from build123d import *

# Parameters (mm, degrees)
BOSS_EXTRUDE1_DEPTH = 3.175
SKETCH2_R           = 1.5875
SKETCH2_W           = 80.264
SKETCH2_H           = 12.954
CUT_EXTRUDE1_DEPTH  = 223.985606318
SKETCH7_R           = 2.032
SKETCH7_R_2         = 1.651
SKETCH7_W           = 47.244
SKETCH7_H           = 139.192
CUT_EXTRUDE4_DEPTH  = 223.985606318
SKETCH8_R           = 1.651
CUT_EXTRUDE5_DEPTH  = 223.985606318
SKETCH9_R           = 1.778
CUT_EXTRUDE6_DEPTH  = 221.482742149
CUT_EXTRUDE7_DEPTH  = 221.482742149


with BuildPart() as part:
    # Sketch1 → Boss-Extrude1 (new body)
    with BuildSketch(Plane(origin=(0, 0, 0), x_dir=(1, 0, 0), z_dir=(0, 1, 0))):
        with BuildLine():
            Line((-80, 112.5), (100, 112.5))
            Line((100, 112.5), (100, -112.5))
            Line((100, -112.5), (-80, -112.5))
            ThreePointArc((-80, -112.5), (-192.5, 0), (-80, 112.5))
        make_face()
    extrude(amount=-BOSS_EXTRUDE1_DEPTH)

    # Sketch2 → Cut-Extrude1 (cut, through all)
    with BuildSketch(Plane(origin=(0, 0, 0), x_dir=(1, 0, 0), z_dir=(0, 1, 0))):
        with Locations(Location((36.144045702, -66.3448, 0), (0, 0, 270))):
            Circle(SKETCH2_R)
        with Locations(Location((36.144045702, -59.9948, 0), (0, 0, 270))):
            Circle(SKETCH2_R)
        with Locations(Location((36.144045702, -53.6448, 0), (0, 0, 270))):
            Circle(SKETCH2_R)
        with Locations(Location((36.144045702, -47.2948, 0), (0, 0, 270))):
            Circle(SKETCH2_R)
        with Locations(Location((36.144045702, -40.9448, 0), (0, 0, 270))):
            Circle(SKETCH2_R)
        with Locations(Location((36.144045702, -34.5948, 0), (0, 0, 270))):
            Circle(SKETCH2_R)
        with Locations(Location((36.144045702, -28.2448, 0), (0, 0, 270))):
            Circle(SKETCH2_R)
        with Locations(Location((67.894045702, -66.3448, 0), (0, 0, 270))):
            Circle(SKETCH2_R)
        with Locations(Location((67.894045702, -59.9948, 0), (0, 0, 270))):
            Circle(SKETCH2_R)
        with Locations(Location((67.894045702, -53.6448, 0), (0, 0, 270))):
            Circle(SKETCH2_R)
        with Locations(Location((67.894045702, -47.2948, 0), (0, 0, 270))):
            Circle(SKETCH2_R)
        with Locations(Location((67.894045702, -40.9448, 0), (0, 0, 270))):
            Circle(SKETCH2_R)
        with Locations(Location((67.894045702, -34.5948, 0), (0, 0, 270))):
            Circle(SKETCH2_R)
        with Locations(Location((67.894045702, -28.2448, 0), (0, 0, 270))):
            Circle(SKETCH2_R)
        with Locations(Location((36.144045702, 66.3448, 0), (0, 0, 270))):
            Circle(SKETCH2_R)
        with Locations(Location((36.144045702, 59.9948, 0), (0, 0, 270))):
            Circle(SKETCH2_R)
        with Locations(Location((36.144045702, 53.6448, 0), (0, 0, 270))):
            Circle(SKETCH2_R)
        with Locations(Location((36.144045702, 47.2948, 0), (0, 0, 270))):
            Circle(SKETCH2_R)
        with Locations(Location((36.144045702, 40.9448, 0), (0, 0, 270))):
            Circle(SKETCH2_R)
        with Locations(Location((36.144045702, 34.5948, 0), (0, 0, 270))):
            Circle(SKETCH2_R)
        with Locations(Location((36.144045702, 28.2448, 0), (0, 0, 270))):
            Circle(SKETCH2_R)
        with Locations(Location((67.894045702, 66.3448, 0), (0, 0, 270))):
            Circle(SKETCH2_R)
        with Locations(Location((67.894045702, 59.9948, 0), (0, 0, 270))):
            Circle(SKETCH2_R)
        with Locations(Location((67.894045702, 53.6448, 0), (0, 0, 270))):
            Circle(SKETCH2_R)
        with Locations(Location((67.894045702, 47.2948, 0), (0, 0, 270))):
            Circle(SKETCH2_R)
        with Locations(Location((67.894045702, 40.9448, 0), (0, 0, 270))):
            Circle(SKETCH2_R)
        with Locations(Location((67.894045702, 34.5948, 0), (0, 0, 270))):
            Circle(SKETCH2_R)
        with Locations(Location((67.894045702, 28.2448, 0), (0, 0, 270))):
            Circle(SKETCH2_R)
        with Locations((52.019045702, -96.4438)):
            Rectangle(SKETCH2_W, SKETCH2_H)
        with Locations((52.019045702, 96.4438)):
            Rectangle(SKETCH2_W, SKETCH2_H)
    extrude(amount=-CUT_EXTRUDE1_DEPTH, mode=Mode.SUBTRACT)

    # Sketch7 → Cut-Extrude4 (cut, through all)
    with BuildSketch(Plane(origin=(0, 0, 0), x_dir=(1, 0, 0), z_dir=(0, 1, 0))):
        with Locations(Location((-50.421540267, 0, 0), (0, 0, 270))):
            Circle(SKETCH7_R)
        with Locations(Location((25.778459733, 0, 0), (0, 0, 270))):
            Circle(SKETCH7_R_2)
        with Locations(Location((86.738459733, 0, 0), (0, 0, 270))):
            Circle(SKETCH7_R_2)
        with Locations(Location((-50.421540267, 40.64, 0), (0, 0, 270))):
            Circle(SKETCH7_R_2)
        with Locations(Location((-50.421540267, -40.64, 0), (0, 0, 270))):
            Circle(SKETCH7_R_2)
        with Locations(Location((15.872459733, -40.64, 0), (0, 0, 270))):
            Circle(SKETCH7_R)
        with Locations(Location((15.872459733, 40.64, 0), (0, 0, 270))):
            Circle(SKETCH7_R)
        with Locations((-14.099540267, 0)):
            Rectangle(SKETCH7_W, SKETCH7_H)
    extrude(amount=-CUT_EXTRUDE4_DEPTH, mode=Mode.SUBTRACT)

    # Sketch8 → Cut-Extrude5 (cut, through all)
    with BuildSketch(Plane(origin=(0, 0, 0), x_dir=(1, 0, 0), z_dir=(0, 1, 0))):
        with Locations(Location((-177.3836, 33.02, 0), (0, 0, 270))):
            Circle(SKETCH8_R)
        with Locations(Location((-177.3836, -33.02, 0), (0, 0, 270))):
            Circle(SKETCH8_R)
        with Locations(Location((-151.9836, 33.02, 0), (0, 0, 270))):
            Circle(SKETCH8_R)
        with Locations(Location((-151.9836, -33.02, 0), (0, 0, 270))):
            Circle(SKETCH8_R)
        with BuildLine():
            Line((-167.0966, 25.4), (-229.776686608, 25.4))
            Line((-229.776686608, 25.4), (-229.776686608, -25.4))
            Line((-229.776686608, -25.4), (-167.0966, -25.4))
            ThreePointArc((-167.0966, -25.4), (-141.6966, 0), (-167.0966, 25.4))
        make_face()
    extrude(amount=-CUT_EXTRUDE5_DEPTH, mode=Mode.SUBTRACT)

    # Sketch9 → Cut-Extrude6 (cut, through all)
    with BuildSketch(Plane(origin=(0, 0, 0), x_dir=(1, 0, 0), z_dir=(0, 1, 0))):
        with Locations(Location((-161.795319669, -55.88, 0), (0, 0, 270))):
            Circle(SKETCH9_R)
        with Locations(Location((-124.964619687, -86.784626771, 0), (0, 0, 270))):
            Circle(SKETCH9_R)
        with Locations(Location((-161.795319669, 55.88, 0), (0, 0, 270))):
            Circle(SKETCH9_R)
        with Locations(Location((-124.964619687, 86.784626771, 0), (0, 0, 270))):
            Circle(SKETCH9_R)
    extrude(amount=-CUT_EXTRUDE6_DEPTH, mode=Mode.SUBTRACT)

    # Sketch10 → Cut-Extrude7 (cut, through all)
    with BuildSketch(Plane(origin=(0, 0, 0), x_dir=(1, 0, 0), z_dir=(0, 1, 0))):
        Polygon((0, 127.979520785), (0, 78.672810993), (20.125086798, 78.672810993), (20.125086798, 17.499658407), (114.992352539, 17.499658407), (114.992352539, -151.143860627), (-214.259658065, -151.143860627), (-214.259658065, 127.979520785), align=None)
    extrude(amount=-CUT_EXTRUDE7_DEPTH, mode=Mode.SUBTRACT)


solid = part.part
Check sheet for the modelled part. Datum: model origin and axes. Units: mm. A direction names the side the tool comes from. Give positions to 0.01 mm unless a question says otherwise; leave off trailing zeros. Loops run counter-clockwise (first coordinate to the right, second up) from the corner with the lowest first, then second, coordinate; pieces in that order, holes last. Notation, with made-up numbers: M -38.5,60 L -26.5,60 A25 cw -26.5,72 Z; hole C 71.25,-2 d9. An arc over 180 degrees is marked long. Return JSON: item names as keys, results as strings. Group by question number.
1. Go/stop test with flat-tipped pins: pin 1 (1.9 mm diameter, centred on x = 36.14, z = -40.94, fed in from +Y); pin 2 (1.6 mm diameter, centred on x = 9, y = -1.5, fed in from +Z). Record where each tip stops, or that it passes through.
2. Cross-section at D-D on z = -56.5. Record the boundary of the cut face in (x, y) (3 decimals).
3. Tool access check on faces 1 (the flat face through (62, -3.175, -66)), 2 (the flat face through (10, -2, -78.673)), 3 (the flat face through (51, -2, -89.967)). Record the directions out of +Z, -Z, +X, -X, +Y, -Y that give a thin tool (end or side, any length) a straight path to the whole face; none if there is none.
4. Thickness scan on L1, parallel to X at y = -0.9, z = -94; L2, parallel to Z at x = 21, y = -2.6; L3, parallel to X at y = -2.4, z = -77. Record the ranges inside material, lowest first.
5. Mould release check, pull along X, two halves, no side actions. Record for faces 4 (the flat face through (49, -2, -112.5)), 5 (the flat face through (100, -2, -66)), 6 (the cylindrical face through (66.486, -1.565, -27.512)): released by +X, released by -X, zero draft, split by the parting line, or undercut.
6. Cross-section at C-C on y = -1.9. State how many separate pieces and enclosed holes the cut face has, plus the area to 3 significant figures.
7. Cross-section at A-A on z = -92. Record the boundary of the cut face in (x, y) (3 decimals), plus the area to 3 significant figures.
8. Cross-section at B-B on x = 86.5. Record the boundary of the cut face in (y, z) (3 decimals).
Return value:
{
 "1": {"pin 1": "through", "pin 2": "z = -78.67"},
 "2": {"outline": "M 20.125,-3.175 L 100,-3.175 L 100,0 L 20.125,0 Z"},
 "3": {"face 1": "+Z, -Z, +X, -X, -Y", "face 2": "+Z, -X, +Y, -Y", "face 3": "+Y, -Y"},
 "4": {"L1": "0 to 11.89, 92.15 to 100", "L2": "-112.5 to -102.92, -89.97 to -17.5", "L3": "20.13 to 100"},
 "5": {"face 4": "zero draft", "face 5": "released by +X", "face 6": "undercut"},
 "6": {"separate pieces": "1", "enclosed holes": "15", "area": "7,120 mm^2"},
 "7": {"outline": "M 0,-3.175 L 11.887,-3.175 L 11.887,0 L 0,0 Z; M 92.151,-3.175 L 100,-3.175 L 100,0 L 92.151,0 Z", "area": "62.7 mm^2"},
 "8": {"outline": "M -3.175,-112.5 L 0,-112.5 L 0,-102.921 L -3.175,-102.921 Z; M -3.175,-89.967 L 0,-89.967 L 0,-17.5 L -3.175,-17.5 Z"}
}
